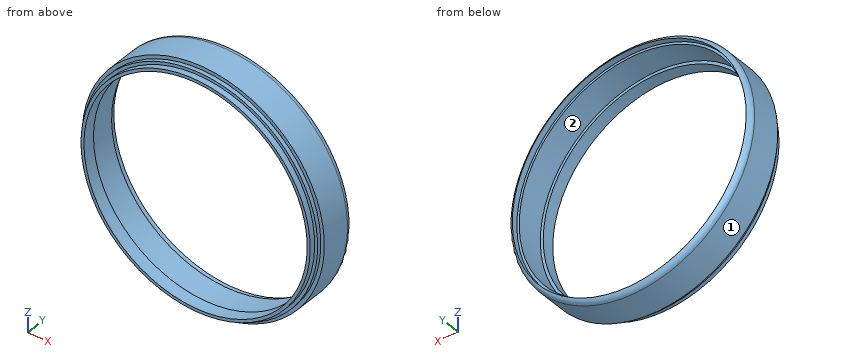
from build123d import *

# Parameters (mm, degrees)
CONG_1_R = 1


with BuildPart() as part:
    # Esquisse1 → Révolution1 (revolve)
    with BuildSketch(Plane.XY, mode=Mode.PRIVATE) as r_volution1_sk:
        Polygon((19, 2.1), (19, 0), (19.5, 0), (19.5, 1), (20, 1), (20, 1.7), (20.6, 1.7), (20.6, 7.75), (19.9, 7.75), (19.9, 6.75), (19.5, 6.75), (19.5, 2.1), align=None)
    revolve(r_volution1_sk.sketch.rotate(Axis((0, 0, 0), (0, 1, 0)), 90), axis=Axis((0, 0, 0), (0, 1, 0)))

    # Congé1
    # the kernel refuses this fillet: 1 mm, written as the material it takes off along each edge
    with BuildSketch(Plane(origin=(0, 7.75, 0), x_dir=(0, 0, -1), z_dir=(1, 0, 0))) as cong_1_piece_1:
        with BuildLine():
            CenterArc((19.6, -0.953939201), CONG_1_R, 0, 72.542396876)
            Line((19.9, 0), (19.906, 0.019078784))
            ThreePointArc((19.906, 0.019078784), (20.25, 0.02), (20.6, 0.02))
            Line((20.6, 0.02), (20.62, 0))
            Line((20.62, 0), (20.62, -0.953939201))
            Line((20.62, -0.953939201), (20.6, -0.953939201))
        make_face()
    revolve(axis=Axis((0, 7.75, 0), (0, 1, 0)), mode=Mode.SUBTRACT)


solid = part.part
The listing builds one solid part. Answer for the finished solid, in the listing's coordinates (mm). Face numbers are marked on the shaded views. Round coordinates to 2 decimals unless told otherwise and drop trailing zeros. Order: outer loops, then holes, each group sorted by start corner. A loop starts at its lowest first (then second) coordinate and runs counter-clockwise, first axis right, second up. Notation, with made-up numbers: (56, 10) -> (113, 10) arc R29 ccw to (113, 43) -> close; hole circle Ø5 at (-34.5, -12.5). An arc over 180 degrees is marked (long way). Put each result on its own line as item: value.
Q1. Section C-C, the plane y = 4 is taken. Write down the section's boundary in (x, z).
Results list:
outline: circle Ø41.2 at (0, 0); hole circle Ø39 at (0, 0)
Q2. Each of these flat-tipped pins is pushed along its axis until it touches: P1, Ø10, axis at x = -7, z = 14.5, coming from the -Y side; P2, Ø1, axis at x = 13, y = 1.5, coming from the +Z side; P3, Ø1.5, axis at y = 6.5, z = 2, coming from the -X side; P4, Ø1, axis at y = 3.5, z = -16.5, coming from the +X side. Where does it stop, or does it pass through?
Results list:
P1: y = 0
P2: z = 16.34
P3: x = -20.56
P4: x = 12.98
Q3. Consider line 1 along X through (y, z) = (3.25, 0); line 2 along X through (y, z) = (1.25, 0); line 3 along Z through (x, y) = (-13, 3). Determine where each line is inside the solid, lowest interval first.
Results list:
line 1: -20.6 to -19.5, 19.5 to 20.6
line 2: -20 to -19, 19 to 20
line 3: -15.98 to -14.53, 14.53 to 15.98
Q4. Section A-A, the plane z = 0 is taken. Write down the section's boundary in (x, y).
Results list:
outline: (-20.6, 1.7) -> (-20, 1.7) -> (-20, 1) -> (-19.5, 1) -> (-19.5, 0) -> (-19, 0) -> (-19, 2.1) -> (-19.5, 2.1) -> (-19.5, 6.75) -> (-19.9, 6.75) -> (-19.9, 7.75) arc R1 ccw to (-20.6, 6.8) -> close; (19, 0) -> (19.5, 0) -> (19.5, 1) -> (20, 1) -> (20, 1.7) -> (20.6, 1.7) -> (20.6, 6.8) arc R1 ccw to (19.9, 7.75) -> (19.9, 6.75) -> (19.5, 6.75) -> (19.5, 2.1) -> (19, 2.1) -> close
Q5. Determine the mould class of the marked faces 1 and 2 for opening direction Z: pulls with the +Z half, pulls with the -Z half, needs draft (parallel to the pull), parting line crosses it, or undercut.
Results list:
face 1: parting line crosses it
face 2: undercut
Q6. Section B-B, the plane x = 0 is taken. Write down the section's boundary in (y, z).
Results list:
outline: (0, -19.5) -> (1, -19.5) -> (1, -20) -> (1.7, -20) -> (1.7, -20.6) -> (6.8, -20.6) arc R1 ccw to (7.75, -19.9) -> (6.75, -19.9) -> (6.75, -19.5) -> (2.1, -19.5) -> (2.1, -19) -> (0, -19) -> close; (0, 19) -> (2.1, 19) -> (2.1, 19.5) -> (6.75, 19.5) -> (6.75, 19.9) -> (7.75, 19.9) arc R1 ccw to (6.8, 20.6) -> (1.7, 20.6) -> (1.7, 20) -> (1, 20) -> (1, 19.5) -> (0, 19.5) -> close
